Source: CAD feature listing. Evaluate the final solid. Frame: model axes, mm. Face numbers are marked on the shaded views. A direction names the side the tool comes from. Round coordinates to 2 decimals unless told otherwise and drop trailing zeros. Order: outer loops, then holes, each group sorted by start corner. A loop starts at its lowest first (then second) coordinate and runs counter-clockwise, first axis right, second up. Notation, with made-up numbers: M 16,-6 L 53,-6 A19 ccw 53,10 Z; hole C -26,58.5 d11. An arc over 180 degrees is marked long. Use one line per item in the form item = value. Start each with the question number.
Q1. Contact query for a flat-ended pin moving along its axis: pin 1 (3 mm diameter, centred on x = -6, y = 1, fed in from +Z). Output: stop coordinate, or through.
Q2. Section C-C (y = 2). Return the cut outline in (x, z).
Q3. Pull-direction query (Y, two-part tool) for the marked faces 1, 2 and 3; classes: pulls with the +Y half, pulls with the -Y half, needs draft (parallel to the pull), parting line crosses it, or undercut.
Q4. Section B-B (z = 1.9). Return the cut outline in (x, y), plus the area to 3 significant figures.
Q5. Reachability of the marked faces 4 and 5 from +Z, -Z, +X, -X, +Y, -Y: full face, straight path, thin tool, end or side. Return the list, or none.
Q6. Material intervals for probe 1 along Y at (x, z) = (0, 1.05); probe 2 along Y at (x, z) = (7, 2.6); probe 3 along X at (y, z) = (-0.75, 3.35), sorted ascending.
Q7. Section A-A (x = 13). Return the cut outline in (y, z).
Q8. Section D-D (x = 0). Return the cut outline in (y, z).
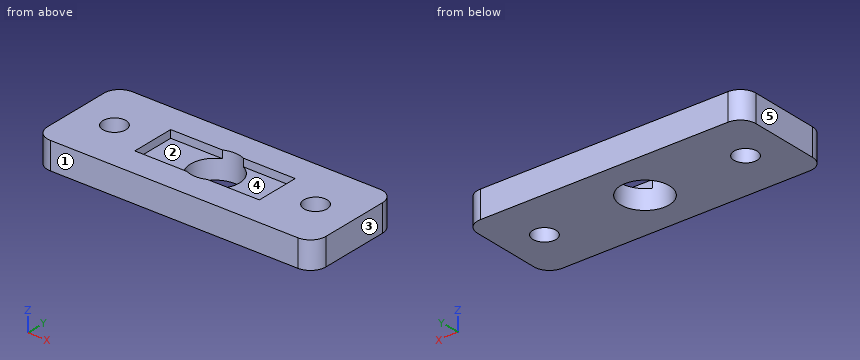
from build123d import *

# Parameters (mm, degrees)
F0_W     = 36
F0_H     = 13
F0_R     = 1.5
F1_DEPTH = 3.5
F2_R     = 2
F4_DEPTH = 1


with BuildPart() as f1:
    # F0 (on Top) → F1 (new body)
    with BuildSketch(Plane.XY):
        Rectangle(F0_W, F0_H)
        with Locations((-13, 0)):
            Circle(F0_R, mode=Mode.SUBTRACT)
        with BuildLine():
            ThreePointArc((3.15, 0), (0, -3.15), (-3.15, 0))
            ThreePointArc((-3.15, 0), (0, 3.15), (3.15, 0))
        make_face(mode=Mode.SUBTRACT)
        with BuildLine():
            ThreePointArc((14.5, 0), (13, -1.5), (11.5, 0))
            ThreePointArc((11.5, 0), (13, 1.5), (14.5, 0))
        make_face(mode=Mode.SUBTRACT)
    extrude(amount=F1_DEPTH)

    # F2
    f2_edges = [f1.edges().sort_by_distance(p)[0] for p in [
        (-18, 6.5, 1.75),
        (-18, -6.5, 1.75),
        (18, -6.5, 1.75),
        (18, 6.5, 1.75),
    ]]
    fillet(f2_edges, radius=F2_R)

    # F3 (on face) → F4 (cut)
    with BuildSketch(Plane.XY.offset(3.5)):
        with BuildLine():
            Line((-1.3416407865, 2.85), (-8.05, 2.85))
            Line((-8.05, 2.85), (-8.05, -2.85))
            Line((-8.05, -2.85), (-1.3416407865, -2.85))
            ThreePointArc((-1.3416407865, -2.85), (-3.15, 0), (-1.3416407865, 2.85))
        make_face()
        with BuildLine():
            Line((1.3416407865, 2.85), (-1.3416407865, 2.85))
            ThreePointArc((-1.3416407865, 2.85), (-3.15, 0), (-1.3416407865, -2.85))
            Line((-1.3416407865, -2.85), (1.3416407865, -2.85))
            ThreePointArc((1.3416407865, -2.85), (2.6597620643, -1.6876509595), (3.15, 0))
            ThreePointArc((3.15, 0), (2.6597620643, 1.6876509595), (1.3416407865, 2.85))
        make_face()
        with BuildLine():
            Line((8.05, 2.85), (1.3416407865, 2.85))
            ThreePointArc((1.3416407865, 2.85), (2.6597620643, 1.6876509595), (3.15, 0))
            ThreePointArc((3.15, 0), (2.6597620643, -1.6876509595), (1.3416407865, -2.85))
            Line((1.3416407865, -2.85), (8.05, -2.85))
            Line((8.05, -2.85), (8.05, 2.85))
        make_face()
    extrude(amount=-F4_DEPTH, mode=Mode.SUBTRACT)


solid = f1.part
Results list:
q1.pin_1 = 2.5
q2.outline = M -18,0 L -2.43,0 L -2.43,2.5 L -8.05,2.5 L -8.05,3.5 L -18,3.5 Z; M 2.43,0 L 18,0 L 18,3.5 L 8.05,3.5 L 8.05,2.5 L 2.43,2.5 Z
q3.face_1 = pulls with the -Y half
q3.face_2 = undercut
q3.face_3 = needs draft
q4.outline = M -18,-4.5 A2 ccw -16,-6.5 L 16,-6.5 A2 ccw 18,-4.5 L 18,4.5 A2 ccw 16,6.5 L -16,6.5 A2 ccw -18,4.5 Z; hole C -13,0 d3; hole C 0,0 d6.3; hole C 13,0 d3
q4.area = 419 mm2
q5.face_4 = +Z
q5.face_5 = +Z, -Z, -X, +Y, -Y
q6.probe_1 = -6.5 to -3.15, 3.15 to 6.5
q6.probe_2 = -6.5 to -2.85, 2.85 to 6.5
q6.probe_3 = -18 to -14.3, -11.7 to -8.05, 8.05 to 11.7, 14.3 to 18
q7.outline = M -6.5,0 L -1.5,0 L -1.5,3.5 L -6.5,3.5 Z; M 1.5,0 L 6.5,0 L 6.5,3.5 L 1.5,3.5 Z
q8.outline = M -6.5,0 L -3.15,0 L -3.15,3.5 L -6.5,3.5 Z; M 3.15,0 L 6.5,0 L 6.5,3.5 L 3.15,3.5 Z
